Work out the finished part from the listing and answer in its coordinate system (mm). Face numbers are marked on the shaded views. A direction names the side the tool comes from. Coordinates: 2 decimals unless noted, no trailing zeros. Loops run counter-clockwise (first coordinate to the right, second up) from the corner with the lowest first, then second, coordinate; pieces in that order, holes last. Notation, with made-up numbers: (46, 11.25) -> (54, 11.25) arc R27 ccw to (54, 27.25) -> close; hole circle Ø8 at (-21, -13). An arc over 180 degrees is marked (long way). Use a Markdown table: item, result. Add a question column.
```python
from build123d import *

# Parameters (mm, degrees)
SKETCH_1_W                = 100
SKETCH_1_H                = 30
EXTRUDE_1_DEPTH           = 20
EXTRUDE_2_DEPTH           = 5
EXTRUDE_2_DEPTH_BACK      = 20
FILLET_1_R                = 5
SKETCH_3_R                = 10
CUT_EXTRUDE_1_DEPTH       = 8
SKETCH_4_R                = 3
CUT_EXTRUDE_2_DEPTH       = 95.599814737
HOLE_WIZARD_1_D           = 5
HOLE_WIZARD_1_CBORE_D     = 10
HOLE_WIZARD_1_CBORE_DEPTH = 6
DRAFT_1_ANGLE             = 5
FILLET_2_R                = 4


with BuildPart() as part:
    # 草图1 → 凸台-拉伸1 (new body)
    with BuildSketch(Plane.XY):
        Rectangle(SKETCH_1_W, SKETCH_1_H)
    extrude(amount=EXTRUDE_1_DEPTH)

    # 草图2 → 凸台-拉伸2 (add, two sides: drawn at the far end of the back side and taken through both)
    with BuildSketch(Plane.XY.offset(20).offset(-EXTRUDE_2_DEPTH_BACK)):
        Polygon((50, -15), (70, -15), (90.695144291, 20.845041382), (50, 20.845041382), align=None)
    extrude(amount=EXTRUDE_2_DEPTH + EXTRUDE_2_DEPTH_BACK)

    # 圆角1
    fillet_1_edges = [part.edges().sort_by_distance(p)[0] for p in [
        (50, 15, 10),
        (50, 0, 20),
    ]]
    fillet(fillet_1_edges, radius=FILLET_1_R - 0.0001)  # a hair under: the kernel refuses the full size

    # 草图3 → 切除-拉伸1 (cut)
    with BuildSketch(Plane.XY.offset(25)):
        with Locations((82.034890253, 15.845041382)):
            Circle(SKETCH_3_R)
    extrude(amount=-CUT_EXTRUDE_1_DEPTH, mode=Mode.SUBTRACT)

    # 草图4 → 切除-拉伸2 (cut, through all)
    with BuildSketch(Plane.XY.offset(17)):
        with Locations((82.034890253, 15.845041382)):
            Circle(SKETCH_4_R)
    extrude(amount=-CUT_EXTRUDE_2_DEPTH, mode=Mode.SUBTRACT)

    # 孔1 (through all)
    with Locations(Plane(origin=(61, 4.845041382, 25), x_dir=(1, 0, 0), z_dir=(0, 0, 1))):
        with Locations((0, 0)):
            CounterBoreHole(HOLE_WIZARD_1_D / 2, HOLE_WIZARD_1_CBORE_D / 2, HOLE_WIZARD_1_CBORE_DEPTH)

    # 拔模1
    draft_1_faces = [part.faces().sort_by_distance(p)[0] for p in [
        (73.374636215, 10.845041382, 21),
    ]]
    draft(draft_1_faces, Plane(origin=(82.034890253, 15.845041382, 17), x_dir=(1, 0, 0), z_dir=(0, 0, 1)), DRAFT_1_ANGLE)

    # 圆角2
    fillet_2_edges = [part.edges().sort_by_distance(p)[0] for p in [
        (90.695144291, 20.845041382, 8.5),
    ]]
    fillet(fillet_2_edges, radius=FILLET_2_R)


solid = part.part
```
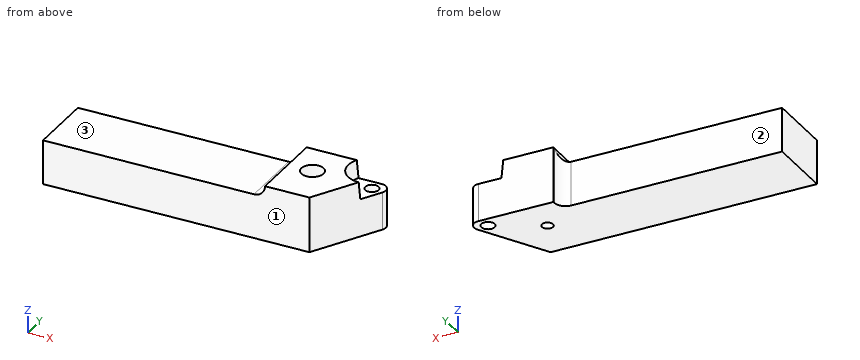
Item 1: Section A-A (x = 61) is taken. Determine the outline of the cut face in (y, z), then the cut area to 3 significant figures.
Item 2: For the marked faces 1, 2 and 3, determine the directions among +Z, -Z, +X, -X, +Y, -Y from which every point of the face is accessible in a straight line to the end or side of a thin tool.
Item 3: Section B-B (z = 8) is taken. Determine the outline of the cut face in (x, y).
Item 4: Find the intervals of material crossed by probe 1 along Y at (x, z) = (61, 11); probe 2 along Y at (x, z) = (11.5, 2.5); probe 3 along Z at (x, y) = (-43.5, -9), in increasing order.
Item 5: Section D-D (z = 22.5) is taken. Determine the outline of the cut face in (x, y).
Item 6: Given pin 1 (9 mm diameter, centred on x = 19.5, y = 2.5, fed in from +Z); pin 2 (1 mm diameter, centred on y = 6, z = 18.5, fed in from +X); pin 3 (3 mm diameter, centred on x = 34, z = 10, fed in from +Y), each flat-ended and moving along its own axis, determine where each tip first touches the part or whether it passes through.
Output:
| question | item | result |
|---|---|---|
| 1 | outline | (-15, 0) -> (2.35, 0) -> (2.35, 19) -> (-0.15, 19) -> (-0.15, 25) -> (-15, 25) -> close; (7.35, 0) -> (20.85, 0) -> (20.85, 25) -> (9.85, 25) -> (9.85, 19) -> (7.35, 19) -> close |
| 1 | area | 741 mm2 |
| 2 | face 1 | +Z, -Z, +X, -X, -Y |
| 2 | face 2 | +Z, -Z, -X, +Y |
| 2 | face 3 | +Z, -X, +Y, -Y |
| 3 | outline | (-50, -15) -> (70, -15) -> (87.23, 14.85) arc R4 ccw to (83.77, 20.85) -> (50, 20.85) -> (50, 20) arc R5 cw to (45, 15) -> (-50, 15) -> close; hole circle Ø5 at (61, 4.85); hole circle Ø6 at (82.03, 15.85) |
| 4 | probe 1 | y = -15 to 2.35, 7.35 to 20.85 |
| 4 | probe 2 | y = -15 to 15 |
| 4 | probe 3 | z = 0 to 20 |
| 5 | outline | (49.33, -15) -> (70, -15) -> (81.76, 5.37) arc R10.48 cw to (72.82, 20.85) -> (50, 20.85) -> (50, 20) arc R5 cw to (49.33, 17.5) -> close; hole circle Ø10 at (61, 4.85) |
| 6 | pin 1 | stops at z = 20 |
| 6 | pin 2 | stops at x = 81.98 |
| 6 | pin 3 | stops at y = 15 |
